The listing builds one solid part. Answer for the finished solid, in the listing's coordinates (mm). Face numbers are marked on the shaded views. A direction names the side the tool comes from. Round coordinates to 2 decimals unless told otherwise and drop trailing zeros. Loops run counter-clockwise (first coordinate to the right, second up) from the corner with the lowest first, then second, coordinate; pieces in that order, holes last. Notation, with made-up numbers: (-24.5, 65.25) -> (4.5, 65.25) arc R24 cw to (4.5, 99.25) -> close; hole circle Ø1 at (10, 57.5). An arc over 180 degrees is marked (long way). Write each question's results on one line, items separated by ' | '. Start each with the question number.
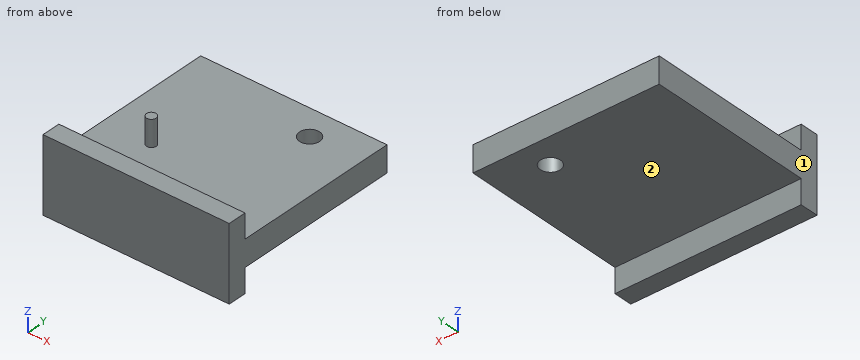
from build123d import *

# Parameters (mm, degrees)
SKETCH_1_W      = 40
SKETCH_1_H      = 50
SKETCH_1_R      = 2.7
EXTRUDE_1_DEPTH = 3.5
SKETCH_3_W      = 40
SKETCH_3_H      = 5
EXTRUDE_2_DEPTH = 10
EXTRUDE_3_DEPTH = 10
SKETCH_5_R      = 1.3
EXTRUDE_4_DEPTH = 7


with BuildPart() as part:
    # 草图1 → 凸台-拉伸1 (new, symmetric)
    with BuildSketch(Plane.XY):
        with Locations((0, 25)):
            Rectangle(SKETCH_1_W, SKETCH_1_H)
        with Locations((6, 42)):
            Circle(SKETCH_1_R, mode=Mode.SUBTRACT)
    extrude(amount=EXTRUDE_1_DEPTH, both=True)

    # 草图3 → 凸台-拉伸2 (add, symmetric)
    with BuildSketch(Plane.XY):
        with Locations((0, 2.5)):
            Rectangle(SKETCH_3_W, SKETCH_3_H)
    extrude(amount=EXTRUDE_2_DEPTH, both=True)

    # 草图7 → 凸台-拉伸3 (add)
    with BuildSketch(Plane.ZY.offset(20)):
        Polygon((-10, 0), (10, 0), (10, 5), (3.5, 5), (3.5, 50), (-3.5, 50), (-3.5, 5), (-10, 5), align=None)
    extrude(amount=EXTRUDE_3_DEPTH)

    # 草图5 → 凸台-拉伸4 (add)
    with BuildSketch(Plane.XY.offset(3.5)):
        with Locations((-17, 19)):
            Circle(SKETCH_5_R)
    extrude(amount=EXTRUDE_4_DEPTH)


solid = part.part
Item 1: For the marked faces 1 and 2, determine the directions among +Z, -Z, +X, -X, +Y, -Y from which every point of the face is accessible in a straight line to the end or side of a thin tool.
Item 2: Each of these flat-tipped pins is pushed along its axis until it touches: pin 1 Ø13.5 at (x, y) = (-3, 25.5) entering from -Z; pin 2 Ø1 at (x, y) = (-13.5, 35) entering from +Z; pin 3 Ø5.5 at (x, y) = (-7.5, 2) entering from +Z. Where does it stop, or does it pass through?
Item 3: The part is cut by section C-C, the plane x = 6. Give the vertices of the cut face in (y, z), plus the area to 3 significant figures.
Item 4: The part is cut by section D-D, the plane y = 19. Give the vertices of the cut face in (x, z), plus the area to 3 significant figures.
Item 5: The part is cut by section B-B, the plane x = -17. Give the vertices of the cut face in (y, z), plus the area to 3 significant figures.
Item 6: Straight lines are drawn through the part: L1, parallel to Y at x = 6, z = 1.75; L2, parallel to Z at x = -3.5, y = 23; L3, parallel to Y at x = -4.5, z = -6.25. For each, find the intervals that lie inside material, in ascending order. Write a range as [from, to].
Item 7: The part is cut by section A-A, the plane y = 42. Give the vertices of the cut face in (x, z), plus the area to 3 significant figures.
Report:
1) face 1: +Z, -Z, -X, +Y, -Y | face 2: -Z, +X, -X, +Y
2) pin 1: stops at z = -3.5 | pin 2: stops at z = 3.5 | pin 3: stops at z = 10
3) outline: (0, -10) -> (5, -10) -> (5, -3.5) -> (39.3, -3.5) -> (39.3, 3.5) -> (5, 3.5) -> (5, 10) -> (0, 10) -> close; (44.7, -3.5) -> (50, -3.5) -> (50, 3.5) -> (44.7, 3.5) -> close | area: 377 mm2
4) outline: (-30, -3.5) -> (20, -3.5) -> (20, 3.5) -> (-15.7, 3.5) -> (-15.7, 10.5) -> (-18.3, 10.5) -> (-18.3, 3.5) -> (-30, 3.5) -> close | area: 368 mm2
5) outline: (0, -10) -> (5, -10) -> (5, -3.5) -> (50, -3.5) -> (50, 3.5) -> (20.3, 3.5) -> (20.3, 10.5) -> (17.7, 10.5) -> (17.7, 3.5) -> (5, 3.5) -> (5, 10) -> (0, 10) -> close | area: 433 mm2
6) L1: y = [0, 39.3], [44.7, 50] | L2: z = [-3.5, 3.5] | L3: y = [0, 5]
7) outline: (-30, -3.5) -> (3.3, -3.5) -> (3.3, 3.5) -> (-30, 3.5) -> close; (8.7, -3.5) -> (20, -3.5) -> (20, 3.5) -> (8.7, 3.5) -> close | area: 312 mm2
